Check sheet for the drawn part. Datum: minimum x, y, z corner. Units: mm. A direction names the side the tool comes from. Give positions to 0.01 mm unless a question says otherwise; leave off trailing zeros. Loops run counter-clockwise (first coordinate to the right, second up) from the corner with the lowest first, then second, coordinate; pieces in that order, holes last. Notation, with made-up numbers: (-19.5, 82) - (-14.5, 82) arc R20 cw to (-14.5, 89) - close; hole circle Ø5 at (84.5, 85). An arc over 180 degrees is marked (long way). Use one line per item in the form item = value.
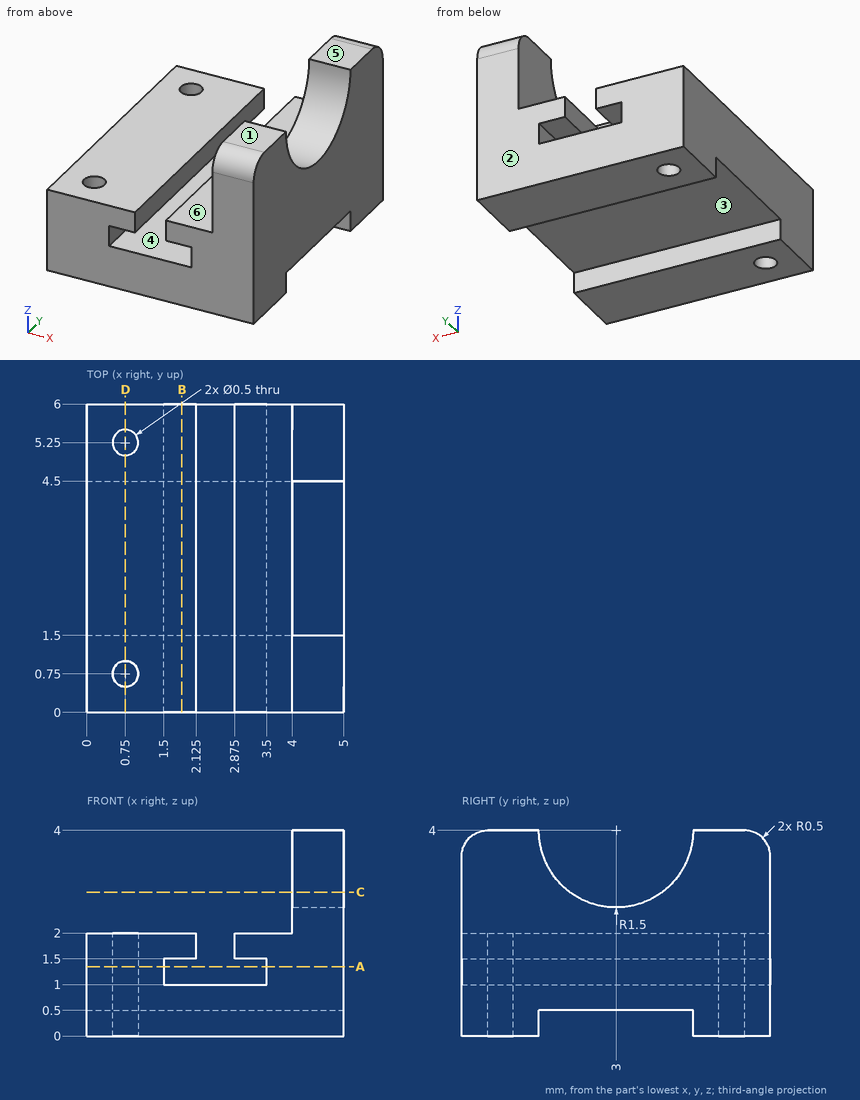
Item 1: Section check A-A on z = 1.35. Record the boundary of the cut face in (x, y), then the cut area to 3 significant figures.
Answer block:
outline = (0, 0) - (1.5, 0) - (1.5, 6) - (0, 6) - close; (3.5, 0) - (5, 0) - (5, 6) - (3.5, 6) - close; hole circle Ø0.5 at (0.75, 0.75); hole circle Ø0.5 at (0.75, 5.25)
area = 17.6 mm2
Item 2: Thickness scan on L1, parallel to X at y = 0.75, z = 1.1; L2, parallel to Y at x = 1.6, z = 0.3; L3, parallel to Z at x = 1.75, y = 1.45. Record the ranges inside material, lowest first.
Answer block:
L1 = 0 to 0.5, 1 to 1.5, 3.5 to 5
L2 = 0 to 1.5, 4.5 to 6
L3 = 0 to 1, 1.5 to 2
Item 3: Access from +Z, -Z, +X, -X, +Y, -Y to the whole of each face (thin tool, end or side, straight path). Record for the marked faces 4, 5 and 6.
Answer block:
face_4 = +Y, -Y
face_5 = +Z, +X, -X, +Y, -Y
face_6 = +Z, -X, +Y, -Y
Item 4: Section check D-D on x = 0.75. Record the boundary of the cut face in (y, z), then the cut area to 3 significant figures.
Answer block:
outline = (0, 0) - (0.5, 0) - (0.5, 2) - (0, 2) - close; (1, 0) - (1.5, 0) - (1.5, 0.5) - (4.5, 0.5) - (4.5, 0) - (5, 0) - (5, 2) - (1, 2) - close; (5.5, 0) - (6, 0) - (6, 2) - (5.5, 2) - close
area = 8.50 mm2
Item 5: Section check B-B on x = 1.85. Record the boundary of the cut face in (y, z), then the cut area to 3 significant figures.
Answer block:
outline = (0, 0) - (1.5, 0) - (1.5, 0.5) - (4.5, 0.5) - (4.5, 0) - (6, 0) - (6, 1) - (0, 1) - close; (0, 1.5) - (6, 1.5) - (6, 2) - (0, 2) - close
area = 7.50 mm2
Item 6: Gauge pin test, flat ends, axial feed: P1, Ø0.9, axis at x = 2, y = 3.5, coming from the -Z side; P2, Ø1, axis at x = 2, z = 3, coming from the -Y side; P3, Ø2, axis at x = 2.5, y = 2, coming from the +Z side. Record the tip position at first contact, or that the pin passes through.
Answer block:
P1 = 0.5
P2 = through
P3 = 2
Item 7: Mould release check, pull along Y, two halves, no side actions. Record for the marked faces 1, 2 and 3: released by +Y, released by -Y, zero draft, split by the parting line, or undercut.
Answer block:
face_1 = zero draft
face_2 = released by +Y
face_3 = undercut
Item 8: Section check C-C on z = 2.8. Record the boundary of the cut face in (x, y).
Answer block:
outline = (4, 0) - (5, 0) - (5, 2.1) - (4, 2.1) - close; (4, 3.9) - (5, 3.9) - (5, 6) - (4, 6) - close
